Work out the finished part from the listing and answer in its coordinate system (mm). A direction names the side the tool comes from. Coordinates: 2 decimals unless noted, no trailing zeros. Write each loop counter-clockwise with the first axis right and the second up, starting at its lowest first coordinate (ties: lowest second). Pieces come first, ordered by that corner, then holes. Notation, with made-up numbers: (70.5, 13.25) - (84.5, 13.25) arc R8 ccw to (84.5, 26.25) - close; hole circle Ø1 at (4, -8.75). An arc over 180 degrees is marked (long way). Use one line per item in the form item = value. Start each with the question number.
Item 1: A cutting plane is placed at D-D (z = -3.75). Write down the section's boundary in (x, y).
Item 2: A cutting plane is placed at A-A (x = 0). Write down the section's boundary in (y, z), then the cut area to 3 significant figures.
Item 3: A cutting plane is placed at C-C (y = 5.5). Write down the section's boundary in (x, z), then the cut area to 3 significant figures.
Item 4: A cutting plane is placed at B-B (z = 0). Write down the section's boundary in (x, y).
Item 5: Given pin 1 (4 mm diameter, centred on x = 7.25, z = -7.25, fed in from -Y); pin 2 (5.5 mm diameter, centred on x = -2, z = 1.5, fed in from +Y); pin 3 (2 mm diameter, centred on x = -2, y = -11, fed in from +Z), each flat-ended and moving along its own axis, determine where each tip first touches the part or whether it passes through.
Item 6: Consider probe 1 along X at (y, z) = (-4, 0); probe 2 along Z at (x, y) = (-0.25, -12); probe 3 along X at (y, z) = (-16.9, 0). Determine where each line is inside the solid, lowest interval first.
Item 7: For faces 1 (the flat face through (2, -18, 2)), 2 (the flat face through (-0.2, 3.5, 8.2)), 3 (the flat face through (-0.2, 0, 8.2)), determine the directions among +Z, -Z, +X, -X, +Y, -Y from which every point of the face is accessible in a straight line to the end or side of a thin tool.
from build123d import *

# Parameters (mm, degrees)
SKETCH1_R           = 12.5
BOSS_EXTRUDE1_DEPTH = 3.5
BOSS_EXTRUDE2_START = 3.5
SKETCH2_R           = 8
SKETCH2_R_2         = 5.5
BOSS_EXTRUDE2_DEPTH = 3.5
SKETCH2_2_R         = 8
SKETCH2_2_R_2       = 5.5
BOSS_EXTRUDE3_DEPTH = 18
SKETCH3_R           = 5.5
CUT_EXTRUDE1_DEPTH  = 8
BOSS_EXTRUDE4_START = -18
SKETCH4_R           = 5.5
SKETCH4_R_2         = 2.05
BOSS_EXTRUDE4_DEPTH = 2.5
SKETCH5_R           = 1.5
CUT_EXTRUDE2_DEPTH  = 8


with BuildPart() as part:
    # Sketch1 → Boss-Extrude1 (new body)
    with BuildSketch(Plane(origin=(0, 0, 0), x_dir=(1, 0, 0), z_dir=(0, 1, 0))):
        Circle(SKETCH1_R)
    extrude(amount=BOSS_EXTRUDE1_DEPTH)

    # Sketch2 → Boss-Extrude2 (add)
    with BuildSketch(Plane(origin=(0, 0, 0), x_dir=(1, 0, 0), z_dir=(0, 1, 0)).offset(BOSS_EXTRUDE2_START)):
        Circle(SKETCH2_R)
        Circle(SKETCH2_R_2, mode=Mode.SUBTRACT)
    extrude(amount=BOSS_EXTRUDE2_DEPTH)

    # Sketch2<2> → Boss-Extrude3 (add)
    with BuildSketch(Plane(origin=(0, 0, 0), x_dir=(1, 0, 0), z_dir=(0, 1, 0))):
        Circle(SKETCH2_2_R)
        Circle(SKETCH2_2_R_2, mode=Mode.SUBTRACT)
    extrude(amount=-BOSS_EXTRUDE3_DEPTH)

    # Sketch3 → Cut-Extrude1 (cut, through all)
    with BuildSketch(Plane(origin=(0, 0, 0), x_dir=(1, 0, 0), z_dir=(0, 1, 0))):
        Circle(SKETCH3_R)
    extrude(amount=CUT_EXTRUDE1_DEPTH, mode=Mode.SUBTRACT)

    # Sketch4 → Boss-Extrude4 (add)
    with BuildSketch(Plane(origin=(0, 0, 0), x_dir=(1, 0, 0), z_dir=(0, 1, 0)).offset(BOSS_EXTRUDE4_START)):
        Circle(SKETCH4_R)
        Circle(SKETCH4_R_2, mode=Mode.SUBTRACT)
    extrude(amount=BOSS_EXTRUDE4_DEPTH)

    # Sketch5 → Cut-Extrude2 (cut, through all)
    with BuildSketch(Plane(origin=(0, 0, 0), x_dir=(1, 0, 0), z_dir=(0, 1, 0))):
        with Locations((-7.247844507, 7.247844507)):
            Circle(SKETCH5_R)
        with Locations((7.247844507, 7.247844507)):
            Circle(SKETCH5_R)
        with Locations((7.247844507, -7.247844507)):
            Circle(SKETCH5_R)
        with Locations((-7.247844507, -7.247844507)):
            Circle(SKETCH5_R)
    extrude(amount=CUT_EXTRUDE2_DEPTH, mode=Mode.SUBTRACT)


solid = part.part
Answer:
q1.outline = (-11.92, 0) - (-7.07, 0) - (-7.07, -18) - (7.07, -18) - (7.07, 0) - (11.92, 0) - (11.92, 3.5) - (7.07, 3.5) - (7.07, 7) - (4.02, 7) - (4.02, -15.5) - (-4.02, -15.5) - (-4.02, 7) - (-7.07, 7) - (-7.07, 3.5) - (-11.92, 3.5) - close
q2.outline = (-18, -8) - (0, -8) - (0, -12.5) - (3.5, -12.5) - (3.5, -8) - (7, -8) - (7, -5.5) - (-15.5, -5.5) - (-15.5, -2.05) - (-18, -2.05) - close; (-18, 2.05) - (-15.5, 2.05) - (-15.5, 5.5) - (7, 5.5) - (7, 8) - (3.5, 8) - (3.5, 12.5) - (0, 12.5) - (0, 8) - (-18, 8) - close
q2.area = 174 mm²
q3.outline = circle Ø16 at (0, 0); hole circle Ø11 at (0, 0)
q3.area = 106 mm²
q4.outline = (-12.5, 0) - (-8, 0) - (-8, -18) - (-2.05, -18) - (-2.05, -15.5) - (-5.5, -15.5) - (-5.5, 7) - (-8, 7) - (-8, 3.5) - (-12.5, 3.5) - close; (2.05, -18) - (8, -18) - (8, 0) - (12.5, 0) - (12.5, 3.5) - (8, 3.5) - (8, 7) - (5.5, 7) - (5.5, -15.5) - (2.05, -15.5) - close
q5.pin_1 = 0
q5.pin_2 = -15.5
q5.pin_3 = 7.94
q6.probe_1 = -8 to -5.5, 5.5 to 8
q6.probe_2 = -8 to -5.49, 5.49 to 8
q6.probe_3 = -8 to -2.05, 2.05 to 8
q7.face_1 = +Z, -Z, +X, -X, -Y
q7.face_2 = +Y
q7.face_3 = -Y
